The drawing under review shows one solid part. Ordinate dimensions are in mm from its lowest x, y, z. Coordinates: 2 decimals unless noted, no trailing zeros. Loops run counter-clockwise (first coordinate to the right, second up) from the corner with the lowest first, then second, coordinate; pieces in that order, holes last.
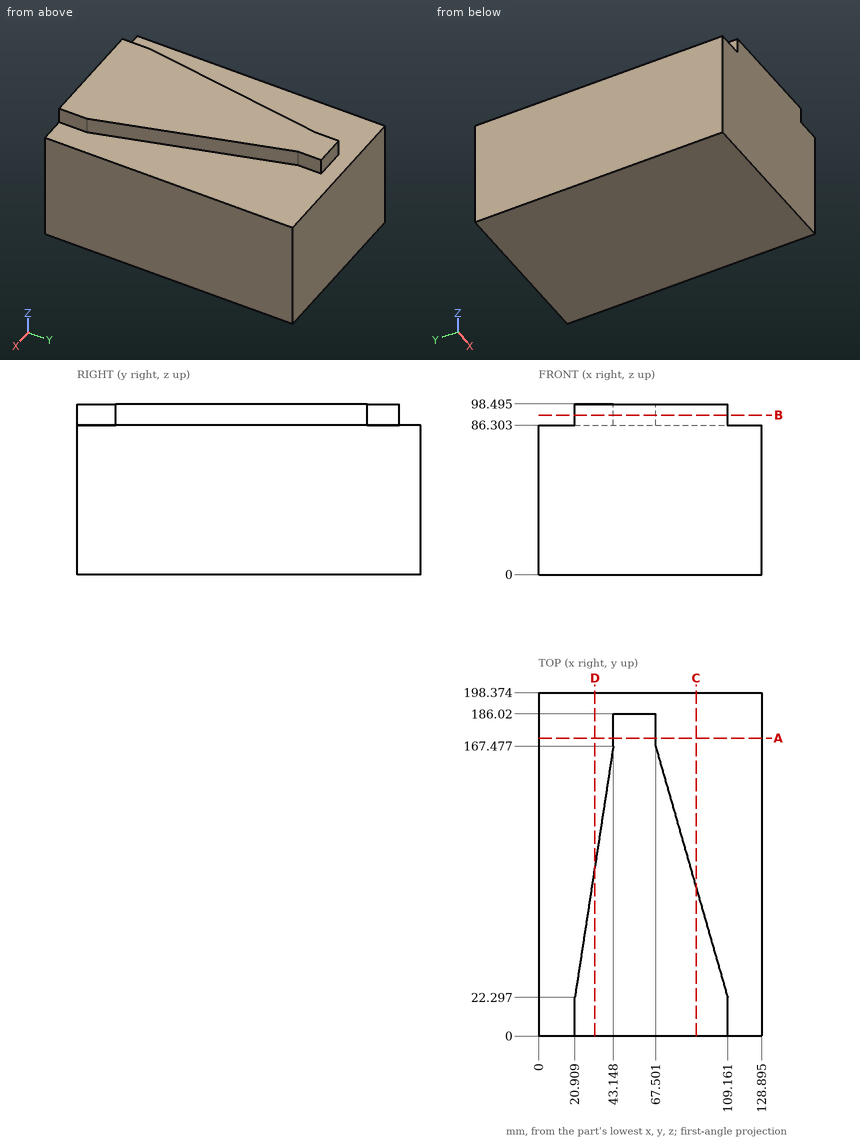
Q1. Take a section at A-A, the plane y = 172. Write out the cut boundary in (x, z) (1 decimal), then the cut area to 3 significant figures.
Q2. Clearance check with flat-ended pins moving along their axes: pin 1 Ø3.5 at (y, z) = (173, 92.5) entering from +X; pin 2 Ø13.5 at (y, z) = (6.5, 94.5) entering from -X; pin 3 Ø3.5 at (y, z) = (173.5, 90.5) entering from -X. State where each tip first meets the part, or that it passes through.
Q3. Take a section at D-D, the plane x = 32.5. Write out the cut boundary in (y, z) (1 decimal), then the cut area to 3 significant figures.
Q4. Take a section at B-B, the plane z = 92. Write out the cut boundary in (x, y).
Q5. For line 1 (Z direction, x = 120, y = 179.5); line 2 (Y direction, x = 49.5, z = 88), list the stretches that pass through material, from the lowest coordinate up.
Q6. Take a section at C-C, the plane x = 91. Write out the cut boundary in (y, z) (1 decimal), then the cut area to 3 significant figures.
Entries:
1. outline: (0, 0) - (128.9, 0) - (128.9, 86.3) - (67.5, 86.3) - (67.5, 98.5) - (43.1, 98.5) - (43.1, 86.3) - (0, 86.3) - close
1. area: 11,400 mm2
2. pin 1: stops at x = 67.5
2. pin 2: stops at x = 20.91
2. pin 3: stops at x = 43.15
3. outline: (0, 0) - (198.4, 0) - (198.4, 86.3) - (98, 86.3) - (98, 98.5) - (0, 98.5) - close
3. area: 18,300 mm2
4. outline: (20.91, 0) - (109.16, 0) - (109.16, 22.3) - (67.5, 167.48) - (67.5, 186.02) - (43.15, 186.02) - (43.15, 167.48) - (20.91, 22.3) - close
5. line 1: z = 0 to 86.3
5. line 2: y = 0 to 186.02
6. outline: (0, 0) - (198.4, 0) - (198.4, 86.3) - (85.6, 86.3) - (85.6, 98.5) - (0, 98.5) - close
6. area: 18,200 mm2
